Verification items for the finished model (mm, model axes). A direction names the side the tool comes from. Give positions to 0.01 mm unless a question says otherwise; leave off trailing zeros. Order: outer loops, then holes, each group sorted by start corner. A loop starts at its lowest first (then second) coordinate and runs counter-clockwise, first axis right, second up. Notation, with made-up numbers: (76.5, 34) -> (88.5, 34) arc R24 cw to (88.5, 71) -> close; hole circle Ø10 at (19, -21). An arc over 180 degrees is marked (long way). Return JSON: item names as keys, results as strings. Group by question number.
(1) Thickness scan on line 1 along Y through (x, z) = (-69, 29); line 2 along Z through (x, y) = (-63.5, 35.5) (3 decimals); line 3 along Y through (x, z) = (-51.5, 218). Record the ranges inside material, lowest first.
(2) Release check for a two-part mould opening along Y. For faces 4 (the face through (-68.87, -24.58, 20.09)), 5 (the face through (-62, 16.566, 216)), 6 (the face through (39, 62, 207.545)) record: pulls with the +Y half, pulls with the -Y half, needs draft (parallel to the pull), parting line crosses it, or undercut.
(3) Cross-section at B-B on z = 152. Enter the section's corners in (x, y), then the cut area to 3 significant figures.
(4) Cross-section at C-C on y = 75. Enter the section's corners in (x, z) (3 decimals), then the cut area to 3 significant figures.
(5) Cross-section at A-A on x = -69.85. State how many separate pieces and enclosed holes the cut face has, then the cut area to 3 significant figures.
(6) Depth check by flat-ended pin: pin 1 Ø8 at (x, z) = (-72, 192.5) entering from +Y; pin 2 Ø5 at (x, z) = (-23.5, 186.5) entering from -Y; pin 3 Ø6 at (x, z) = (-107.5, 131) entering from -Y. Enter the tip coordinate at first touch or a pass-through.
(7) Tool access check on faces 1 (the face through (-69, -25, 55.145)), 2 (the face through (-82, 51, 80.545)), 3 (the face through (-68.87, 146.61, 20.09)). Record the directions out of +Z, -Z, +X, -X, +Y, -Y that give a thin tool (end or side, any length) a straight path to the whole face; none if there is none.
Solid Edge part; units mm, degrees
sketch "Sketch1" plane through (0, 0, 0) normal (1, 0, 0) x (0, 1, 0)
  line L0 (-65.9842, 55.145) -> (61.0158, 55.145)
  line L1 (188.0158, 55.145) -> (61.0158, 55.145)
  line L2 (188.0158, 10.695) -> (188.0158, 55.145)
  line L3 (175.3158, 10.695) -> (188.0158, 10.695)
  line L4 (168.6119, 17.3988) -> (175.3158, 10.695)
  line L5 (156.2658, 29.745) -> (168.6119, 17.3988)
  line L6 (137.2158, 10.695) -> (156.2658, 29.745)
  line L7 (-15.1842, 10.695) -> (137.2158, 10.695)
  line L8 (-15.1842, 10.695) -> (-34.2342, 29.745)
  line L9 (-34.2342, 29.745) -> (-53.2842, 10.695)
  line L10 (-53.2842, 10.695) -> (-65.9842, 10.695)
  line L11 (-65.9842, 10.695) -> (-65.9842, 55.145)
extrude "Protrusion1" add sketch "Sketch1" against normal blind 139.7
sketch "Sketch2" plane through (0, 0, 0) normal (1, 0, 0) x (0, 1, 0)
  line L0 (16.5658, 207.545) -> (16.5658, 55.145)
  line L1 (16.5658, 55.145) -> (105.4658, 55.145)
  line L2 (105.4658, 55.145) -> (105.4658, 207.545)
  line L3 (105.4658, 207.545) -> (16.5658, 207.545)
extrude "ExtrudedProtrusion_2" add sketch "Sketch2" against normal blind 139.7
sketch "Sketch3" plane through (0, 0, 0) normal (1, 0, 0) x (0, 1, 0)
  line L0 (16.5658, 207.545) -> (16.5658, 283.745)
  line L1 (16.5658, 283.745) -> (105.4658, 283.745)
  line L2 (105.4658, 283.745) -> (105.4658, 207.545)
  line L3 (105.4658, 207.545) -> (16.5658, 207.545)
extrude "ExtrudedProtrusion_3" add sketch "Sketch3" against normal blind 203.2 and the other way blind 76.2
sketch "Sketch4" plane through (-63.5, 16.5658, 169.445) normal (0, -1, 0) x (1, 0, 0)
  line L0 (31.75, 38.1) -> (31.75, -88.9)
  line L1 (31.75, -88.9) -> (-76.2, -88.9)
  line L2 (-76.2, -88.9) -> (-76.2, 38.1)
  line L3 (-76.2, 38.1) -> (31.75, 38.1)
extrude "ExtrudedCutout_2" cut sketch "Sketch4" against normal blind 63.5 and the other way through all
sketch "Sketch5" plane through (76.2, 61.0158, 245.645) normal (1, 0, 0) x (0, 1, 0)
  circle A0 centre (0, 0) radius 19.05
extrude "Cutout1" cut sketch "Sketch5" against normal through all and the other way through all
fillet "Round_1" radius 6.35 16 edges at (-31.75, 16.5658, 144.045) (-85.725, 16.5658, 80.545) (-69.85, 16.5658, 55.145) (-117.475, 16.5658, 207.545) (38.1, 16.5658, 207.545) (-139.7, 80.0658, 144.045) (-139.7, 48.3158, 80.545) (-69.85, -65.9842, 55.145) (38.1, 105.4658, 207.545) (-63.5, 105.4658, 283.745) (-63.5, 16.5658, 283.745) (-171.45, 105.4658, 207.545) (-69.85, 105.4658, 55.145) (-69.85, 188.0158, 55.145) (-69.85, 188.0158, 10.695) (-69.85, -65.9842, 10.695)
sketch "Sketch6" plane through (-69.85, 61.0158, 10.695) normal (0, 0, -1) x (-1, 0, 0)
  circle A0 centre (0, 0) radius 9.525
extrude "Cutout2" cut sketch "Sketch6" against normal up to next and the other way through all
Verdict:
{
 "1": {"line 1": "-65.98 to -34.98, -33.49 to 51.53, 70.5 to 155.52, 157.01 to 188.02", "line 2": "10.695 to 80.545, 207.545 to 283.745", "line 3": "16.57 to 105.47"},
 "2": {"face 4": "undercut", "face 5": "pulls with the -Y half", "face 6": "needs draft"},
 "3": {"outline": "(-139.7, 86.42) arc R6.35 ccw to (-133.35, 80.07) -> (-31.75, 80.07) -> (-31.75, 22.92) arc R6.35 ccw to (-25.4, 16.57) -> (0, 16.57) -> (0, 105.47) -> (-139.7, 105.47) -> close", "area": "5,550 mm²"},
 "4": {"outline": "(-203.2, 207.545) -> (-31.75, 207.545) -> (-31.75, 80.545) -> (-133.35, 80.545) arc R6.35 ccw to (-139.7, 74.195) -> (-139.7, 10.695) -> (0, 10.695) -> (0, 207.545) -> (76.2, 207.545) -> (76.2, 232.709) -> (-203.2, 232.709) -> close; (-203.2, 258.581) -> (76.2, 258.581) -> (76.2, 283.745) -> (-203.2, 283.745) -> close", "area": "27,800 mm²"},
 "5": {"separate pieces": "2", "enclosed holes": "1", "area": "20,300 mm²"},
 "6": {"pin 1": "y = 105.47", "pin 2": "y = 16.57", "pin 3": "y = 80.07"},
 "7": {"face 1": "+Z, +X, -X, -Y", "face 2": "-X, -Y", "face 3": "-Z, +X, -X"}
}
